from build123d import *

# Parameters (mm, degrees)
F1_DEPTH    = 508
F2_T1_DEPTH = 192.0875
F3_R        = 3.175
F4_DEPTH    = 1.5875
F5_R        = 3.175
F6_DEPTH    = 1.5875


# Not quite as in the source:
# - a fillet or chamfer that OpenCascade refuses, or shapes differently, is made with other operations: its cross-section is extruded or revolved along the edge and cut away or added


with BuildPart() as f1:
    # F0 (on Top) → F1 (new body)
    with BuildSketch(Plane.XY):
        Polygon((-11.3587090754, 18.7056229889), (-12.9462090754, 18.7056229889), (-12.9462090754, -19.3943770111), (25.1537909246, -19.3943770111), (25.1537909246, -17.8068770111), (-11.3587090754, -17.8068770111), align=None)
    extrude(amount=F1_DEPTH)

    # F2: fillet of radius 38.1 on 2 edges, made by hand

    # F2_s2 → F2_t1 (cut)
    with BuildSketch(Plane.YZ.offset(-108.1962090754)):
        with BuildLine():
            add(Edge.make_bspline(
                [(18.7056229889, 469.9), (18.7056229889, 508), (-19.3943770111, 508)],
                knots=[0, 0, 0, 1, 1, 1], degree=2, weights=[1, 1, 1]))
            Line((-19.3943770111, 508), (18.7056229889, 508))
            Line((18.7056229889, 508), (18.7056229889, 469.9))
        make_face()
        with BuildLine():
            add(Edge.make_bspline(
                [(18.7056229889, 38.1), (18.7056229889, 0), (-19.3943770111, 0)],
                knots=[0, 0, 0, 1, 1, 1], degree=2, weights=[1, 1, 1]))
            Line((-19.3943770111, 0), (18.7056229889, 0))
            Line((18.7056229889, 0), (18.7056229889, 38.1))
        make_face()
    extrude(amount=F2_T1_DEPTH, mode=Mode.SUBTRACT)

    # F3 (on face) → F4 (cut)
    with BuildSketch(Plane(origin=(-12.9462090754, 0, 0), x_dir=(0, -1, 0), z_dir=(-1, 0, 0))):
        with Locations((0.3443770111, 488.9331097904)):
            Circle(F3_R)
        with Locations((0.3443770111, 19.0668902096)):
            Circle(F3_R)
    extrude(amount=-F4_DEPTH, mode=Mode.SUBTRACT)

    # F5 (on face) → F6 (cut)
    with BuildSketch(Plane.XZ.offset(19.3943770111)):
        with Locations((6.1037909246, 12.7)):
            Circle(F5_R)
        with Locations((6.1037909246, 495.3)):
            Circle(F5_R)
    extrude(amount=-F6_DEPTH, mode=Mode.SUBTRACT)


solid = f1.part
Could you check a few things on this model? Use its own coordinates, in mm. A direction names the side the tool comes from. Give positions to 0.01 mm unless a question says otherwise; leave off trailing zeros. Write each loop counter-clockwise with the first axis right and the second up, starting at its lowest first coordinate (ties: lowest second). Pieces come first, ordered by that corner, then holes. Notation, with made-up numbers: (52, -30) -> (70, -30) arc R27 ccw to (70, -4) -> close; hole circle Ø10 at (49, 82.25). An arc over 180 degrees is marked (long way). Write each question's results on one line, items separated by ' | '. Start each with the question number.
Q1. Suppose I cut it at A-A, the plane z = 117. List the corners of the cut face in (x, y) for me.
Q2. Which directions (+Z, -Z, +X, -X, +Y, -Y) give clear straight access to the entire face, cutting with the end or side of a thin tool? Please do faces 1 (the face through (-12.946, 0, 250)), 2 (the face through (-11.359, 0, 250)).
Q3. I'm going to push flat-ended pins straight in: pin 1 Ø18.5 at (x, z) = (-2, 278.5) entering from +Y; pin 2 Ø3 at (y, z) = (12, 61) entering from +X. Where does each tip first touch, or does it pass through?
Q4. I need wall thicknesses on probe 1 along X at (y, z) = (-19, 495.3); probe 2 along Y at (x, z) = (-10, 124); probe 3 along X at (y, z) = (-7, 159.5). Which ranges of each line are inside material? Lowest first, please.
Outcome:
1) outline: (-12.95, -19.39) -> (25.15, -19.39) -> (25.15, -17.81) -> (-11.36, -17.81) -> (-11.36, 18.71) -> (-12.95, 18.71) -> close
2) face 1: +Z, -Z, -X, +Y, -Y | face 2: +Z, -Z, +X, +Y
3) pin 1: y = -17.81 | pin 2: x = -11.36
4) probe 1: -12.95 to 2.93, 9.28 to 25.15 | probe 2: -19.39 to -17.81 | probe 3: -12.95 to -11.36
